```python
from build123d import *

# Parameters (mm, degrees)
BOSS_EXTRUDE1_DEPTH         = 12.7
F_1_4_20_TAPPED_HOLE2_D     = 5.1054
F_1_4_20_TAPPED_HOLE2_DEPTH = 19.05
F_1_4_20_TAPPED_HOLE2_TIP   = 1.533816902


with BuildPart() as part:
    # Sketch1 → Boss-Extrude1 (new body)
    with BuildSketch(Plane(origin=(0, 0, 0), x_dir=(1, 0, 0), z_dir=(0, 1, 0))):
        with BuildLine():
            Line((25.4, 0), (165.1, 0))
            ThreePointArc((165.1, 0), (183.060512242, 7.439487758), (190.5, 25.4))
            Line((190.5, 25.4), (190.5, 177.8))
            ThreePointArc((190.5, 177.8), (183.060512242, 195.760512242), (165.1, 203.2))
            Line((165.1, 203.2), (25.4, 203.2))
            ThreePointArc((25.4, 203.2), (7.439487758, 195.760512242), (0, 177.8))
            Line((0, 177.8), (0, 25.4))
            ThreePointArc((0, 25.4), (7.439487758, 7.439487758), (25.4, 0))
        make_face()
    extrude(amount=BOSS_EXTRUDE1_DEPTH)

    # 1/4-20 Tapped Hole2
    with Locations(Plane(origin=(0, 12.7, 0), x_dir=(1, 0, 0), z_dir=(0, 1, 0))):
        with Locations((95.25, 151.6), (95.25, 51.6)):
            Hole(F_1_4_20_TAPPED_HOLE2_D / 2, depth=F_1_4_20_TAPPED_HOLE2_DEPTH)
            with Locations((0, 0, -(F_1_4_20_TAPPED_HOLE2_DEPTH + F_1_4_20_TAPPED_HOLE2_TIP / 2))):  # 118° drill point
                Cone(0, F_1_4_20_TAPPED_HOLE2_D / 2, F_1_4_20_TAPPED_HOLE2_TIP, mode=Mode.SUBTRACT)


solid = part.part
```
Model file for the job. Use its own axes, mm. Coordinates: 2 decimals unless noted, no trailing zeros. Loops run counter-clockwise (first coordinate to the right, second up) from the corner with the lowest first, then second, coordinate; pieces in that order, holes last. Notation, with made-up numbers: (-34.5, 12) - (-10.5, 12) arc R22 ccw to (-10.5, 26) - close; hole circle Ø10 at (68.5, 25). An arc over 180 degrees is marked (long way). Answer as a JSON object with one key per item and string values. Group by question number.
(1) Cut at B-B (z = -51.6). Give the cut face in (x, y), then the cut area to 3 significant figures.
(2) Cut at C-C (y = 2). Give the cut face in (x, z), then the cut area to 3 significant figures.
(3) Two-plate mould, pull along X, no slides. Class faces 1 (the face through (94, 12.7, -103)), 2 (the face through (182.86, 6.26, -7.24)), 3 (the face through (95.803, 6.261, -49.108)): released by +X, released by -X, zero draft, split by the parting line, or undercut.
(4) Cut at A-A (x = 95.25). Give the cut face in (y, z).
(5) Probe line 1 along Z through (x, y) = (95.25, 4); line 2 along X through (y, z) = (2.5, -151.6); line 3 along Z through (x, y) = (169, 1). List the from-to ranges inside material, lowest first.
Geometry says:
{
 "1": {"outline": "(0, 0) - (92.7, 0) - (92.7, 12.7) - (0, 12.7) - close; (97.8, 0) - (190.5, 0) - (190.5, 12.7) - (97.8, 12.7) - close", "area": "2,350 mm^2"},
 "2": {"outline": "(0, -177.8) arc R25.4 ccw to (25.4, -203.2) - (165.1, -203.2) arc R25.4 ccw to (190.5, -177.8) - (190.5, -25.4) arc R25.4 ccw to (165.1, 0) - (25.4, 0) arc R25.4 ccw to (0, -25.4) - close; hole circle Ø5.11 at (95.25, -151.6); hole circle Ø5.11 at (95.25, -51.6)", "area": "38,100 mm^2"},
 "3": {"face 1": "zero draft", "face 2": "released by +X", "face 3": "undercut"},
 "4": {"outline": "(0, -203.2) - (12.7, -203.2) - (12.7, -154.15) - (0, -154.15) - close; (0, -149.05) - (12.7, -149.05) - (12.7, -54.15) - (0, -54.15) - close; (0, -49.05) - (12.7, -49.05) - (12.7, 0) - (0, 0) - close"},
 "5": {"line 1": "z = -203.2 to -154.15, -149.05 to -54.15, -49.05 to 0", "line 2": "x = 0 to 92.7, 97.8 to 190.5", "line 3": "z = -202.9 to -0.3"}
}
